```python
from build123d import *

# Parameters (mm, degrees)
EXTRUDE1_DEPTH        = 152.4
EXTRUDE2_DEPTH        = 3.175
SKETCH8_R             = 3.175
EXTRUDE4_DEPTH        = 191.248536063
LPATTERN1_COUNT       = 5
LPATTERN1_PITCH       = 37.30625
MIRROR5_COPY_1_DEPTH  = 3.175
MIRROR5_COPY_2_DEPTH  = 3.175
MIRROR5_COPY_3_DEPTH  = 3.175
MIRROR5_COPY_4_DEPTH  = 3.175
EXTRUDE5_DEPTH        = 25.4
EXTRUDE_THIN2_START   = -23.563494
SKETCH12_R            = 26.9875
SKETCH12_R_2          = 22.225
EXTRUDE_THIN2_DEPTH   = 23.563494
EXTRUDE_THIN2_2_DEPTH = 23.563494
SKETCH13_W            = 17.78
SKETCH13_H            = 5.08
SKETCH13_W_2          = 5.08
SKETCH13_H_2          = 13.97
SKETCH13_H_3          = 20.32
SKETCH13_W_3          = 19.05
SKETCH13_W_4          = 16.51
SKETCH13_H_4          = 12.685889217
SKETCH13_W_5          = 15.24
EXTRUDE6_DEPTH        = 23.563494
FILLET1_R             = 3.302


with BuildPart() as part:
    # Sketch1 → Extrude1 (new body)
    with BuildSketch(Plane.XY):
        Polygon((39.132231405, 0), (112.500773126, 0), (112.500773126, 5.890873545), (87.100773126, 5.890873545), (87.100773126, 23.563494179), (39.132231405, 23.563494179), align=None)
    extrude1 = extrude(amount=-EXTRUDE1_DEPTH)

    # Mirror1: Extrude1 across plane
    add(extrude1.mirror(Plane(origin=(39.132231405, 23.563494179, -152.4), x_dir=(0, 0, 1), z_dir=(-1, 0, 0))))

    # Sketch6 → Extrude2 (add)
    with BuildSketch(Plane.XY):
        Polygon((87.100773126, 23.563494179), (112.500773126, 5.890873545), (87.100773126, 5.890873545), align=None)
    extrude2 = extrude(amount=-EXTRUDE2_DEPTH)

    # Sketch8 → Extrude4 (cut, through all)
    with BuildSketch(Plane(origin=(0, 5.890873545, 0), x_dir=(-1, 0, 0), z_dir=(0, 1, 0))):
        with Locations((-100.395913074, -19.446875)):
            Circle(SKETCH8_R)
        with Locations((-100.395913074, -56.753125)):
            Circle(SKETCH8_R)
        with Locations((-100.395913074, -95.518958881)):
            Circle(SKETCH8_R)
        with Locations((-100.395913074, -132.953125)):
            Circle(SKETCH8_R)
    extrude4 = extrude(amount=-EXTRUDE4_DEPTH, mode=Mode.SUBTRACT)

    # LPattern1: Extrude2 ×5
    with Locations(*[(0, 0, -i * LPATTERN1_PITCH) for i in range(1, LPATTERN1_COUNT)]):
        add(extrude2)

    # Mirror5: Extrude2, Extrude4 across plane
    add(extrude2.mirror(Plane(origin=(39.132231405, 0, 0), x_dir=(0, 0, 1), z_dir=(1, 0, 0))))
    add(extrude4.mirror(Plane(origin=(39.132231405, 0, 0), x_dir=(0, 0, 1), z_dir=(1, 0, 0))), mode=Mode.SUBTRACT)

    # Mirror5 copy 1 sketch → Mirror5 copy 1 (add)
    with BuildSketch(Plane(origin=(78.264462809, 0, -37.30625), x_dir=(-1, 0, 0), z_dir=(0, 0, 1))):
        Polygon((87.100773126, -23.563494179), (112.500773126, -5.890873545), (87.100773126, -5.890873545), align=None)
    extrude(amount=-MIRROR5_COPY_1_DEPTH)

    # Mirror5 copy 2 sketch → Mirror5 copy 2 (add)
    with BuildSketch(Plane(origin=(78.264462809, 0, -74.6125), x_dir=(-1, 0, 0), z_dir=(0, 0, 1))):
        Polygon((87.100773126, -23.563494179), (112.500773126, -5.890873545), (87.100773126, -5.890873545), align=None)
    extrude(amount=-MIRROR5_COPY_2_DEPTH)

    # Mirror5 copy 3 sketch → Mirror5 copy 3 (add)
    with BuildSketch(Plane(origin=(78.264462809, 0, -111.91875), x_dir=(-1, 0, 0), z_dir=(0, 0, 1))):
        Polygon((87.100773126, -23.563494179), (112.500773126, -5.890873545), (87.100773126, -5.890873545), align=None)
    extrude(amount=-MIRROR5_COPY_3_DEPTH)

    # Mirror5 copy 4 sketch → Mirror5 copy 4 (add)
    with BuildSketch(Plane(origin=(78.264462809, 0, -149.225), x_dir=(-1, 0, 0), z_dir=(0, 0, 1))):
        Polygon((87.100773126, -23.563494179), (112.500773126, -5.890873545), (87.100773126, -5.890873545), align=None)
    extrude(amount=-MIRROR5_COPY_4_DEPTH)

    # Sketch11 → Extrude5 (cut)
    with BuildSketch(Plane(origin=(0, 23.563494179, 0), x_dir=(-1, 0, 0), z_dir=(0, 1, 0))):
        with BuildLine():
            Line((-80.750773126, -139.7), (-80.750773126, -12.7))
            ThreePointArc((-80.750773126, -12.7), (-78.890901187, -8.209871939), (-74.400773126, -6.35))
            Line((-74.400773126, -6.35), (-3.863689683, -6.35))
            ThreePointArc((-3.863689683, -6.35), (0.626438378, -8.209871939), (2.486310317, -12.7))
            Line((2.486310317, -12.7), (2.486310317, -139.7))
            ThreePointArc((2.486310317, -139.7), (0.626438378, -144.190128061), (-3.863689683, -146.05))
            Line((-3.863689683, -146.05), (-74.400773126, -146.05))
            ThreePointArc((-74.400773126, -146.05), (-78.890901187, -144.190128061), (-80.750773126, -139.7))
        make_face()
    extrude(amount=-EXTRUDE5_DEPTH, mode=Mode.SUBTRACT)



with BuildPart() as body_2:
    # Sketch12 → Extrude-Thin2 (new body)
    with BuildSketch(Plane(origin=(0, 23.563494179, 0), x_dir=(-1, 0, 0), z_dir=(0, 1, 0)).offset(EXTRUDE_THIN2_START)):
        with Locations((-39.132231405, -41.275)):
            Circle(SKETCH12_R)
        with Locations((-39.132231405, -41.275)):
            Circle(SKETCH12_R_2, mode=Mode.SUBTRACT)
    extrude(amount=EXTRUDE_THIN2_DEPTH)


with BuildPart() as body_3:
    # Sketch12 → Extrude-Thin2 2 (new body)
    with BuildSketch(Plane(origin=(0, 23.563494179, 0), x_dir=(-1, 0, 0), z_dir=(0, 1, 0)).offset(EXTRUDE_THIN2_START)):
        with Locations((-39.132231405, -111.125)):
            Circle(SKETCH12_R)
        with Locations((-39.132231405, -111.125)):
            Circle(SKETCH12_R_2, mode=Mode.SUBTRACT)
    extrude(amount=EXTRUDE_THIN2_2_DEPTH)


with BuildPart() as part_1:
    add(part.part)

    add(body_2.part)  # Extrude6 merges body 2

    add(body_3.part)  # Extrude6 merges body 3
    # Sketch13 → Extrude6 (add)
    with BuildSketch(Plane(origin=(0, 23.563494179, 0), x_dir=(-1, 0, 0), z_dir=(0, 1, 0))):
        with Locations((-71.860773126, -41.275)):
            Rectangle(SKETCH13_W, SKETCH13_H)
        with Locations((-39.132231405, -9.8425)):
            Rectangle(SKETCH13_W_2, SKETCH13_H_2)
        with Locations((-39.132231405, -76.5175)):
            Rectangle(SKETCH13_W_2, SKETCH13_H_3)
        with Locations((-5.159731405, -41.275)):
            Rectangle(SKETCH13_W_3, SKETCH13_H)
        with Locations((-5.337623018, -111.125)):
            Rectangle(SKETCH13_W_4, SKETCH13_H)
        with Locations((-39.132231405, -142.266392139)):
            Rectangle(SKETCH13_W_2, SKETCH13_H_4)
        with Locations((-73.130773126, -111.125)):
            Rectangle(SKETCH13_W_5, SKETCH13_H)
    extrude(amount=-EXTRUDE6_DEPTH)

    # Fillet1
    fillet1_edges = [part_1.edges().sort_by_distance(p)[0] for p in [
        (36.592231405, 11.781747179, -6.35),
        (41.672231405, 11.781747179, -6.35),
        (36.592231405, 11.781747179, -14.407295292),
        (41.672231405, 11.781747179, -14.407295292),
        (36.592231405, 11.781747179, -68.142704708),
        (36.592231405, 11.781747179, -84.257295292),
        (41.672231405, 11.781747179, -84.257295292),
        (41.672231405, 11.781747179, -137.992704708),
        (36.592231405, 11.781747179, -137.992704708),
        (12.264526697, 11.781747179, -108.585),
        (12.264526697, 11.781747179, -113.665),
        (65.999936112, 11.781747179, -113.665),
        (65.999936112, 11.781747179, -108.585),
        (80.750773126, 11.781747179, -113.665),
        (80.750773126, 11.781747179, -108.585),
        (12.264526697, 11.781747179, -38.735),
        (12.264526697, 11.781747179, -43.815),
        (65.999936112, 11.781747179, -43.815),
        (80.750773126, 11.781747179, -43.815),
        (65.999936112, 11.781747179, -38.735),
        (80.750773126, 11.781747179, -38.735),
    ]]
    fillet(fillet1_edges, radius=FILLET1_R)


solid = part_1.part
```
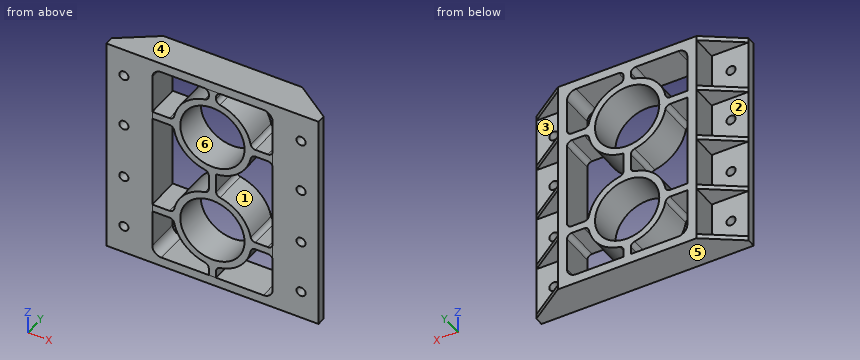
Can you work these out from the model? Positions are in its coordinate system, mm. Face numbers are marked on the shaded views. A direction names the side the tool comes from. Coordinates: 2 decimals unless noted, no trailing zeros. Loops run counter-clockwise (first coordinate to the right, second up) from the corner with the lowest first, then second, coordinate; pieces in that order, holes last. Notation, with made-up numbers: M 58,-19.5 L 109,-19.5 A34 ccw 109,12.5 Z; hole C 20.25,55.25 d3. An arc over 180 degrees is marked long. Put each result on its own line as item: value. Start each with the question number.
(1) Will these pins go through, and if not, where does the flat tip stop? pin 1 Ø11.5 at (y, z) = (15, -125) entering from -X; pin 2 Ø12.5 at (x, z) = (95, -86.5) entering from +Y; pin 3 Ø5 at (x, z) = (14.5, -58) entering from +Y; pin 4 Ø1 at (y, z) = (13, -66.5) entering from +X.
(2) Imagine slicing it at B-B on x = 19. List the corners of the cut face in (y, z) for me.
(3) Imagine slicing it at C-C on z = -87. List the corners of the cut face in (x, y) for me.
(4) We'd pull the mould along Z, two halves only. Please class the marked faces 4, 5 and 6: +Z half, -Z half, draft (parallel to the pull), parting line (faces both ways), or undercut.
(5) Imagine slicing it at D-D on x = -14.5. List the corners of the cut face in (y, z) for me (1 decimal), and give its area (3 significant figures).
(6) Imagine slicing it at A-A on z = -122.5. List the corners of the cut face in (x, y) for me, and give its area (3 significant figures).
(7) I need wall thicknesses on probe 1 along Z at (x, y) = (-22.5, 10.75) (1 decimal); probe 2 along X at (y, z) = (18.25, -105.5); probe 3 along Z at (x, y) = (76.5, 18.5) (3 decimals). Which ranges of each line are inside material? Lowest first, please.
(8) Which directions (+Z, -Z, +X, -X, +Y, -Y) give clear straight access to the entire face, cutting with the end or side of a thin tool? Please do the marked faces 1, 2 and 3.
Worked answers:
1. pin 1: stops at x = -8.84
1. pin 2: stops at y = 5.89
1. pin 3: passes through
1. pin 4: stops at x = 87.1
2. outline: M 0,-152.4 L 23.56,-152.4 L 23.56,-146.05 L 0,-146.05 Z; M 0,-129.1 L 23.56,-129.1 L 23.56,-120.54 L 0,-120.54 Z; M 0,-101.71 L 23.56,-101.71 L 23.56,-93.15 L 0,-93.15 Z; M 0,-59.25 L 23.56,-59.25 L 23.56,-50.69 L 0,-50.69 Z; M 0,-31.86 L 23.56,-31.86 L 23.56,-23.3 L 0,-23.3 Z; M 0,-6.35 L 23.56,-6.35 L 23.56,0 L 0,0 Z
3. outline: M -34.24,0 L -2.49,0 L -2.49,23.56 L -8.84,23.56 L -8.84,5.89 L -34.24,5.89 Z; M 27.04,0 L 51.23,0 L 51.23,23.56 L 27.04,23.56 Z; M 80.75,0 L 112.5,0 L 112.5,5.89 L 87.1,5.89 L 87.1,23.56 L 80.75,23.56 Z
4. face 4: +Z half
4. face 5: -Z half
4. face 6: undercut
5. outline: M 0,-152.4 L 19.6,-152.4 L 19.6,-149.2 L 5.9,-149.2 L 5.9,-115.1 L 19.6,-115.1 L 19.6,-111.9 L 5.9,-111.9 L 5.9,-77.8 L 19.6,-77.8 L 19.6,-74.6 L 5.9,-74.6 L 5.9,-40.5 L 19.6,-40.5 L 19.6,-37.3 L 5.9,-37.3 L 5.9,-3.2 L 19.6,-3.2 L 19.6,0 L 0,0 Z
5. area: 1,120 mm2
6. outline: M -34.24,0 L -2.49,0 L -2.49,23.56 L -8.84,23.56 L -8.84,5.89 L -34.24,5.89 Z; M 14.66,0 L 20.04,0 L 20.04,23.56 L 14.66,23.56 Z; M 58.23,0 L 63.61,0 L 63.61,23.56 L 58.23,23.56 Z; M 80.75,0 L 112.5,0 L 112.5,5.89 L 87.1,5.89 L 87.1,23.56 L 80.75,23.56 Z
6. area: 852 mm2
7. probe 1: z = -152.4 to -149.2, -115.1 to -111.9, -77.8 to -74.6, -40.5 to -37.3, -3.2 to 0
7. probe 2: x = -8.84 to -2.49, 12.74 to 17.63, 60.63 to 65.53, 80.74 to 87.1
7. probe 3: z = -152.4 to -145.693, -113.665 to -108.585, -43.815 to -38.735, -6.707 to 0
8. face 1: +Y, -Y
8. face 2: -X, +Y
8. face 3: +X, +Y
